Design review of the part built by this model. Coordinates are the model's own, in mm. Give positions to 0.01 mm unless a question says otherwise; leave off trailing zeros. Loops run counter-clockwise (first coordinate to the right, second up) from the corner with the lowest first, then second, coordinate; pieces in that order, holes last. Notation, with made-up numbers: (56.25, -37) - (92.25, -37) arc R23 cw to (92.25, -17) - close; hole circle Ø7 at (70.25, 83.25). An arc over 180 degrees is marked (long way). Write each question's results on one line, items separated by ' | '.
Autodesk Fusion 360 part; units mm, degrees
sketch "Sketch1" plane through (0, 0, 0) normal (0, 1, 0) x (1, 0, 0)
  circle A0 centre (0, 0) radius 50
  circle A1 centre (0, 0) radius 30 construction
  circle A2 centre (0, 0) radius 10
  circle A3 centre (0, 0) radius 45
  circle A4 centre (0, 0) radius 40 construction
  line L0 (25, -37.4166) -> (25, 37.4166)
  point P0 (-30, 0)
  point P1 (15, -25.9808)
  point P2 (15, 25.9808)
  point P3 (-40, 0)
  point P4 (20, -34.641)
  point P5 (20, 34.641)
  dimension "d1" = 100
  dimension "d2" = 60
  dimension "d3" = 20
  dimension "d4" = -5
  dimension "d6" = 360
  dimension "d14" = 80
  dimension "d18" = 5
extrude "Extrude1" add sketch "Sketch1" along normal blind 5 contours A3 L0 picked at (20, 0)
hole "Hole1" at (15, 0, 25.9808) at (15, 0, -25.9808) at (-30, 0, 0) direction (0, 1, 0) diameter 4.5 depth 7 tip angle 118
hole "Hole2" at (-40, 0, 0) at (20, 0, 34.641) at (20, 0, -34.641) direction (0, 1, 0) diameter 4.234 depth 25 tip angle 118
Item 1: We need section A-A on x = 0. Give the boundary of the cut face in (y, z).
Output values:
outline: (0, -45) - (5, -45) - (5, -10) - (0, -10) - close; (0, 10) - (5, 10) - (5, 45) - (0, 45) - close
Item 2: We need section D-D on y = 1.85. Give the boundary of the cut face in (x, z), then the cut area to 3 significant figures.
Output values:
outline: (25, -37.42) - (25, 37.42) arc R45 ccw (long way) to start; hole circle Ø4.23 at (-40, 0); hole circle Ø4.5 at (-30, 0); hole circle Ø20 at (0, 0); hole circle Ø4.5 at (15, -25.98); hole circle Ø4.5 at (15, 25.98); hole circle Ø4.23 at (20, -34.64); hole circle Ø4.23 at (20, 34.64) | area: 4,900 mm²
Item 3: We need section C-C on x = 20. Give the boundary of the cut face in (y, z).
Output values:
outline: (0, -40.31) - (5, -40.31) - (5, -36.76) - (0, -36.76) - close; (0, -32.52) - (5, -32.52) - (5, 32.52) - (0, 32.52) - close; (0, 36.76) - (5, 36.76) - (5, 40.31) - (0, 40.31) - close
Item 4: We need section B-B on z = 6. Give the boundary of the cut face in (x, y).
Output values:
outline: (-44.6, 0) - (-8, 0) - (-8, 5) - (-44.6, 5) - close; (8, 0) - (25, 0) - (25, 5) - (8, 5) - close
Item 5: Wall thickness on probe 1 along X at (y, z) = (3.1, 0); probe 2 along Z at (x, y) = (13.5, 0.35); probe 3 along Z at (x, y) = (15, 3.7): over which ranges is each line inside the solid? List them lowest first.
Output values:
probe 1: x = -45 to -42.12, -37.88 to -32.25, -27.75 to -10, 10 to 25 | probe 2: z = -42.93 to -27.66, -24.3 to 24.3, 27.66 to 42.93 | probe 3: z = -42.43 to -28.23, -23.73 to 23.73, 28.23 to 42.43
Item 6: Draft analysis for pull direction X (two halves, no side actions). For faces 1 (the face through (25, 2, 1)), 2 (the face through (-10.5, 0, -0.6)), 3 (the face through (19.36, 2.54, -36.66)), state which applies: +X half, -X half, draft (parallel to the pull), parting line (faces both ways), or undercut.
Output values:
face 1: +X half | face 2: draft | face 3: undercut
Item 7: Clearance check with flat-ended pins moving along their axes: P1, Ø2, axis at x = 10, y = 2.5, coming from the -Z side; P2, Ø3, axis at x = 1, y = 1, coming from the +Z side; P3, Ø4, axis at x = 15, z = -25.98, coming from the -Y side; P4, Ø5.5, axis at x = 20, z = -34.641, coming from the +Y side. State where each tip first meets the part, or that it passes through.
Output values:
P1: stops at z = -44.09 | P2: stops at z = 45 | P3: passes through | P4: stops at y = 5
